The listing builds one solid part. Answer for the finished solid, in the listing's coordinates (mm). A direction names the side the tool comes from. Round coordinates to 2 decimals unless told otherwise and drop trailing zeros. Loops run counter-clockwise (first coordinate to the right, second up) from the corner with the lowest first, then second, coordinate; pieces in that order, holes last. Notation, with made-up numbers: M 23,44 L 29,44 A21 cw 29,66 Z; hole C 70.5,-0.5 d4. An arc over 180 degrees is marked long. Answer as a JSON object with one key per item and string values.
Autodesk Inventor part; units mm, degrees
ref_plane "YZ Plane" through (0, 0, 0) normal (1, 0, 0) x (0, 1, 0)
ref_plane "XZ Plane" through (0, 0, 0) normal (0, 1, 0) x (-1, 0, 0)
ref_plane "XY Plane" through (0, 0, 0) normal (0, 0, 1) x (1, 0, 0)
sketch "スケッチ1" plane through (0, 0, 0) normal (0, 0, 1) x (1, 0, 0)
  circle A0 centre (-18, 0) radius 31.5
  line L0 (0, 0) -> (-18, 0) construction
  circle A1 centre (-36.7, 0) radius 1.5
  circle A2 centre (-36.7, 0) radius 4 construction
  circle A3 centre (-36.7, 0) radius 4.5
  circle A4 centre (-8.65, -16.1947) radius 4.5
  circle A5 centre (-8.65, -16.1947) radius 4 construction
  circle A6 centre (-8.65, -16.1947) radius 1.5
  circle A7 centre (-8.65, 16.1947) radius 4.5
  circle A8 centre (-8.65, 16.1947) radius 4 construction
  circle A9 centre (-8.65, 16.1947) radius 1.5
  circle A10 centre (-18, 0) radius 22
  line L1 (-36.7, 0) -> (-18, 0) construction
  circle A11 centre (-18, 0) radius 22.7 construction
  circle A12 centre (-36.7, 0) radius 2
  circle A13 centre (-8.65, -16.1947) radius 2
  circle A14 centre (-8.65, 16.1947) radius 2
  circle A15 centre (-1.9799, 1.9799) radius 2.8
  circle A16 centre (-1.9799, 1.9799) radius 1.5
  circle A17 centre (-1.9799, -1.9799) radius 1.5
  circle A18 centre (-1.9799, -1.9799) radius 2.8
  circle A19 centre (1.9799, -1.9799) radius 1.5
  circle A20 centre (1.9799, -1.9799) radius 2.8
  circle A21 centre (1.9799, 1.9799) radius 1.5
  circle A22 centre (1.9799, 1.9799) radius 2.8
  line L2 (0, 0) -> (-1.9799, 1.9799)
  point P0 (-1.5877, 1.6905)
  point P1 (-5.0591, 12.5113)
  point P2 (1.2886, 2.8639)
  point P3 (1.2886, -2.8639)
  point P4 (-5.0591, -12.5113)
  point P5 (-13.6354, -17.4628)
  point P6 (-35.3056, -4.9515)
  point P7 (-35.3056, 4.9515)
  point P8 (-13.6354, 17.4628)
  point P9 (0.5827, -2.75)
  point P10 (-4.16, 16.8432)
  point P11 (-4.16, -16.8432)
  point P12 (-10.3333, -20.4074)
  point P13 (-39.5067, -3.5642)
  point P14 (-39.5067, 3.5642)
  point P15 (-10.3333, 20.4074)
  point P16 (-0.2113, 2.75)
  point P17 (-35.9375, 1.4987)
  point P18 (-35.9375, -1.4987)
  point P19 (-7.7333, -14.785)
  point P20 (-10.3292, -16.2837)
  point P21 (-10.3292, 16.2837)
  point P22 (-7.7333, 14.785)
  point P23 (4, 0.041)
  point P24 (4, -0.041)
  point P25 (3.5801, -4.2776)
  point P26 (-4.2595, -17.1813)
  point P27 (-9.9908, -20.4903)
  point P28 (-39.7497, -3.3089)
  point P29 (-39.7497, 3.3089)
  point P30 (-9.9908, 20.4903)
  point P31 (-4.2595, 17.1813)
  point P32 (3.5801, 4.2776)
  dimension "d10" = 63
  dimension "d13" = 3
  dimension "d14" = 8
  dimension "d15" = 9
  dimension "d16" = 360
  dimension "d19" = 9.5
  dimension "d23" = 4
  dimension "d24" = 360
  dimension "d25" = 5.6
  dimension "d26" = 3
  dimension "d30" = 360
  dimension "d46" = 45
  dimension "d47" = 18
  dimension "d49" = 44
  dimension "d50" = 18.7
  dimension "d53" = 0.7
  dimension "d69" = 45.4
extrude "押し出し1" add sketch "スケッチ1" along normal blind 0.8 contours A0 | A3 A10 | A10 A3 | A10 A7 | A7 A10 | A10 A4 | A4 A10 | A22 A10 | A10 A20
extrude "押し出し2" add sketch "スケッチ1" along normal blind 1.5 contours A12 | A13 | A14
extrude "押し出し3" add sketch "スケッチ1" along normal blind 4 contours A1 | A3 A10 A7 A22 A15 A18 A20 A4 | A10 A22 A20 A21 A15 | A20 A18 A19 A22 A10 | A10 A20 A22 | A22 A16 A18 A15 | A15 A21 A22 A16 | A20 A17 A18 A19 | A18 A15 A17 A20 | A22 A19 A20 A21 | A18 A16 A15 A17 | A21 A20 A15 | A22 L2 A16 | A18 A22 A19 | A17 A15 A20 | A18 A16 L2 | A6 | A9 picked at (0.5491, 0.5309) picked at (0.5491, -0.5309) picked at (-0.5491, -0.5309)
sketch "スケッチ2" plane through (0, 0, 4) normal (0, 0, 1) x (1, 0, 0)
  arc A0 (-39.7497, -3.3089) -> (-39.7497, 3.3089) centre (-36.7, 0) ccw
  arc A1 (-39.7497, -3.3089) -> (-9.9908, -20.4903) centre (-18, 0) ccw
  arc A2 (-4.2595, -17.1813) -> (-9.9908, -20.4903) centre (-8.65, -16.1947) ccw
  arc A3 (-4.2595, -17.1813) -> (-4.2595, 17.1813) centre (-18, 0) ccw
  arc A4 (-9.9908, 20.4903) -> (-4.2595, 17.1813) centre (-8.65, 16.1947) ccw
  arc A5 (-9.9908, 20.4903) -> (-39.7497, 3.3089) centre (-18, 0) ccw
  circle A6 centre (1.9799, 1.9799) radius 1.5
  circle A7 centre (-1.9799, -1.9799) radius 1.5
  circle A8 centre (-1.9799, 1.9799) radius 1.5
  circle A9 centre (1.9799, -1.9799) radius 1.5
  arc A10 (-36.9155, -6.4964) -> (-36.9155, 6.4964) centre (-36.7, 0) ccw
  arc A11 (-36.9155, -6.4964) -> (-14.1683, -19.6295) centre (-18, 0) ccw
  arc A12 (-2.9162, -13.1331) -> (-14.1683, -19.6295) centre (-8.65, -16.1947) ccw
  arc A13 (-2.9162, -13.1331) -> (-2.9162, 13.1331) centre (-18, 0) ccw
  arc A14 (-14.1683, 19.6295) -> (-2.9162, 13.1331) centre (-8.65, 16.1947) ccw
  arc A15 (-14.1683, 19.6295) -> (-36.9155, 6.4964) centre (-18, 0) ccw
  circle A16 centre (-1.9799, 1.9799) radius 3.5
  circle A17 centre (-1.9799, -1.9799) radius 3.5
  line L0 (-36.7, 0) -> (0, 0) construction
  line L1 (-36.7, -1) -> (0, -1)
  line L2 (0, 1) -> (-36.7, 1)
  arc A18 (-36.7, 1) -> (-36.7, -1) centre (-36.7, 0) ccw
  arc A19 (0, -1) -> (0, 1) centre (0, 0) ccw
  line L3 (-8.65, 16.1947) -> (-18.35, 0) construction
  line L4 (-9.5079, 16.7085) -> (-19.2079, 0.5138)
  line L5 (-17.4921, -0.5138) -> (-7.7921, 15.6808)
  arc A20 (-7.7921, 15.6808) -> (-9.5079, 16.7085) centre (-8.65, 16.1947) ccw
  arc A21 (-19.2079, 0.5138) -> (-17.4921, -0.5138) centre (-18.35, 0) ccw
  line L6 (-18.35, 0) -> (-8.65, -16.1947) construction
  line L7 (-19.2079, -0.5138) -> (-9.5079, -16.7085)
  line L8 (-7.7921, -15.6808) -> (-17.4921, 0.5138)
  arc A22 (-17.4921, 0.5138) -> (-19.2079, -0.5138) centre (-18.35, 0) ccw
  arc A23 (-9.5079, -16.7085) -> (-7.7921, -15.6808) centre (-8.65, -16.1947) ccw
  circle A24 centre (-0.0604, 6.1052) radius 1.05
  circle A25 centre (-0.0604, -6.1052) radius 1.05
  point P0 (-13.5, 8.0973)
  point P1 (-13.5, -8.0973)
  point P2 (0.9336, -6.4435)
  point P3 (-0.5034, -5.1532)
  point P4 (-5.3399, -1)
  point P5 (-16.5854, -1)
  point P6 (-11.0923, -10.171)
  point P7 (-0.5034, 5.1532)
  point P8 (0.9336, 6.4435)
  point P9 (-11.0923, 10.171)
  point P10 (-16.5854, 1)
  point P11 (-5.3399, 1)
  point P12 (-12.8081, -11.1986)
  point P13 (-18.9167, -1)
  point P14 (-30.2774, -1)
  point P15 (-30.2774, 1)
  point P16 (-18.9167, 1)
  point P17 (-12.8081, 11.1986)
  dimension "d58" = 2
  dimension "d59" = 2
  dimension "d60" = 2
  dimension "d61" = 2
  dimension "d62" = 2
  dimension "d63" = 2
  dimension "d64" = 2.1
  dimension "d65" = 2.1
extrude "押し出し4" cut sketch "スケッチ2" against normal blind 4 contours L1 L7 A12 A11 A10 | A10 A15 A14 L4 L2 | L8 L1 A17 A25 A13 A12 | L5 A14 A13 A24 A16 L2 | A25 | A24
fillet "フィレット1" radius 1.05 18 edges at (-30.2774, 1, 2) (-36.9155, 6.4964, 2) (-14.1683, 19.6295, 2) (-12.8081, 11.1986, 2) (-18.9167, 1, 2) (-18.9167, -1, 2) (-30.2774, -1, 2) (-36.9155, -6.4964, 2) (-14.1683, -19.6295, 2) (-12.8081, -11.1986, 2) (-2.9162, -13.1331, 2) (-11.0923, -10.171, 2) (-16.5854, -1, 2) (-5.3399, 1, 2) (-5.3399, -1, 2) (-11.0923, 10.171, 2) (-2.9162, 13.1331, 2) (-16.5854, 1, 2)
properties part number "クランク4t" material "アルミニウム 7075"
Item 1: Straight lines are drawn through the part: line 1 (Y direction, x = -8.65, z = 2.75); line 2 (X direction, y = 15, z = 2); line 3 (Y direction, x = -22, z = 2.85). For each, find the intervals that lie inside material, in ascending order.
Values follow:
{"line 1": "-17.69 to -14.69, -11.69 to -9.69, -1 to 1, 9.69 to 11.69, 14.69 to 17.69", "line 2": "-34.09 to -31.23, -15.04 to -12.99, -9.56 to -7.74, -4.31 to -1.91", "line 3": "-21.63 to -19.6, -1 to 1, 19.6 to 21.63"}
Item 2: The part is cut by section A-A (x = -8.65). Give the number of separate pieces and of enclosed holes in the cut face, then the cut area to 3 significant figures.
Values follow:
{"separate pieces": "3", "enclosed holes": "0", "area": "74.0 mm^2"}
Item 3: Determine the mould class of faces 4 (the face through (-29.24, 18.91, 2.38)), 5 (the face through (-6.74, 9.98, 2.03)), 6 (the face through (-15, -14.8, 2)), 7 (the face through (-18, 0, 0)) for opening direction X: released by +X, released by -X, zero draft, split by the parting line, or undercut.
Values follow:
{"face 4": "split by the parting line", "face 5": "undercut", "face 6": "undercut", "face 7": "zero draft"}
Item 4: Flat-ended cylindrical pins translate along their axes: P1, Ø1.2, axis at x = -26.5, z = 1.5, coming from the -Y side; P2, Ø1.5, axis at x = 6.5, y = 13, coming from the +Z side; P3, Ø2, axis at y = -10, z = 1.5, coming from the +X side; P4, Ø3.5, axis at x = -1.98, y = 1.98, coming from the -Z side. Find the tip coordinate at first contact, or state that the pin passes through.
Values follow:
{"P1": "y = -20.53", "P2": "z = 0.8", "P3": "x = 12.1", "P4": "z = 0"}
Item 5: The part is cut by section C-C (x = 7.5). Give the vertices of the cut face in (y, z).
Values follow:
{"outline": "M -18.49,0 L 18.49,0 L 18.49,0.8 L -18.49,0.8 Z"}
Item 6: Which of the six approach directions +Z, -Z, +X, -X, +Y, -Y give full straight-line access (tool end or side, diameter ignored) to faces 1 (the face through (-9, 16, 4)), 2 (the face through (-28.156, -17.23, 2.028)), 3 (the face through (-7, -16, 1.5))?
Values follow:
{"face 1": "+Z, +X, -X, +Y, -Y", "face 2": "+Z, -Z", "face 3": "+Z"}
